Design review of the part shown in the three views and the two pictorial views. Dimensions are in mm from the part's minimum x, y and z. A direction names the side the tool comes from. Coordinates: 2 decimals unless noted, no trailing zeros. Loops run counter-clockwise (first coordinate to the right, second up) from the corner with the lowest first, then second, coordinate; pieces in that order, holes last. Notation, with made-up numbers: (-9, 24.5) -> (5, 24.5) arc R5 cw to (5, 33.5) -> close; hole circle Ø5 at (-29, -38). An arc over 180 degrees is marked (long way). Use CSV: the item, a comma, the result in double quotes.
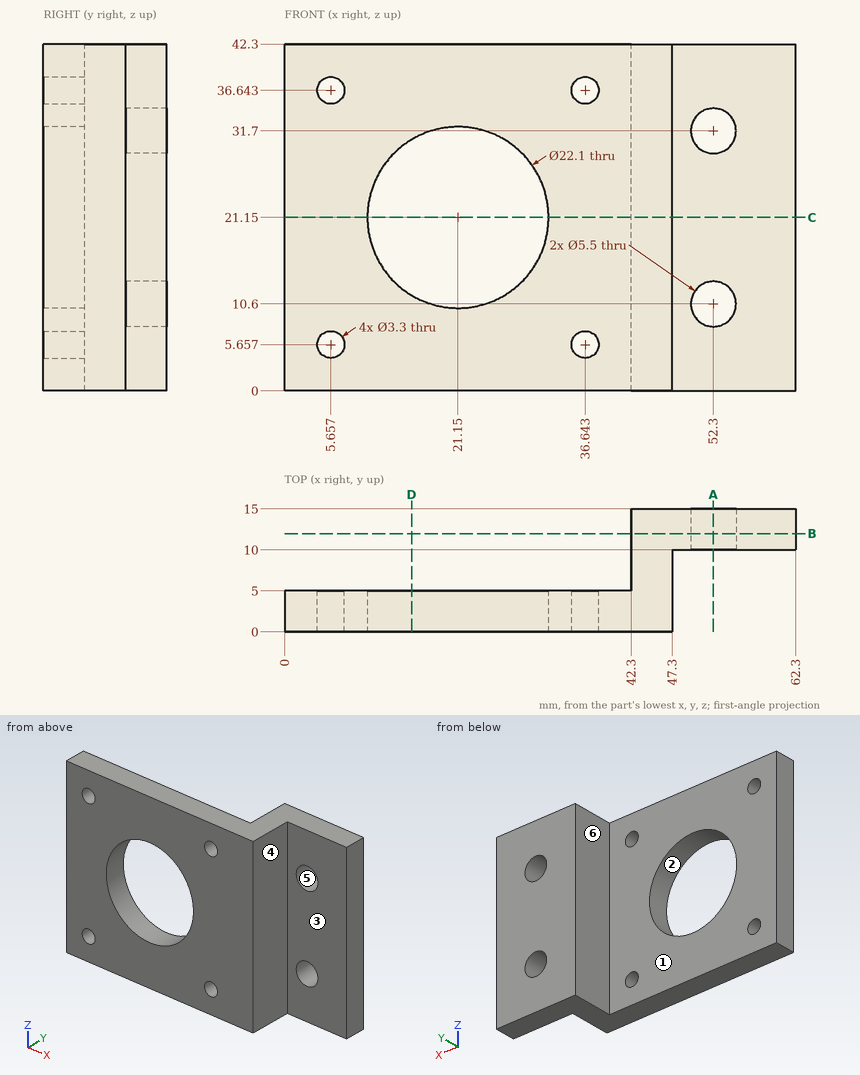
Item 1: Draft analysis for pull direction X (two halves, no side actions). For the marked faces 4, 5 and 6, state which applies: pulls with the +X half, pulls with the -X half, needs draft (parallel to the pull), parting line crosses it, or undercut.
Checked values:
face 4,"pulls with the +X half"
face 5,"undercut"
face 6,"pulls with the -X half"
Item 2: Add section C-C (z = 21.15). Give the boundary of the cut face in (x, y), then the cut area to 3 significant figures.
Checked values:
outline,"(0, 0) -> (10.1, 0) -> (10.1, 5) -> (0, 5) -> close; (32.2, 0) -> (47.3, 0) -> (47.3, 10) -> (62.3, 10) -> (62.3, 15) -> (42.3, 15) -> (42.3, 5) -> (32.2, 5) -> close"
area,"251 mm^2"
Item 3: Machinability: for the marked faces 1, 2 and 3, which of the approach directions +Z, -Z, +X, -X, +Y, -Y give a long, thin tool a straight path to every point of the face, cutting with its end or side? Answer none if there is none.
Checked values:
face 1,"+Z, -Z, -X, +Y"
face 2,"+Y, -Y"
face 3,"+Z, -Z, +X, -Y"
Item 4: Add section B-B (y = 12). Give the boundary of the cut face in (x, z).
Checked values:
outline,"(42.3, 0) -> (62.3, 0) -> (62.3, 42.3) -> (42.3, 42.3) -> close; hole circle Ø5.5 at (52.3, 10.6); hole circle Ø5.5 at (52.3, 31.7)"
Item 5: Add section A-A (x = 52.3). Give the boundary of the cut face in (y, z), then the cut area to 4 significant figures.
Checked values:
outline,"(10, 0) -> (15, 0) -> (15, 7.85) -> (10, 7.85) -> close; (10, 13.35) -> (15, 13.35) -> (15, 28.95) -> (10, 28.95) -> close; (10, 34.45) -> (15, 34.45) -> (15, 42.3) -> (10, 42.3) -> close"
area,"156.5 mm^2"
Item 6: Clearance check with flat-ended pins moving along their axes: pin 1 (5 mm diameter, centred on y = 4, z = 22.5, fed in from +X); pin 2 (8 mm diameter, centred on y = 9.5, z = 14.5, fed in from -X); pin 3 (2.5 mm diameter, centred on x = 5.66, z = 5.66, fed in from -Y); pin 4 (12 mm diameter, centred on x = 54.5, z = 17.5, fed in from -Y). State where each tip first meets the part, or that it passes through.
Checked values:
pin 1,"x = 47.3"
pin 2,"x = 42.3"
pin 3,"through"
pin 4,"y = 10"
Item 7: To check wall thickness, follow line 1 along Z through (x, y) = (52.3, 13.9); line 2 along X through (y, z) = (13.9, 31.7); line 3 along Y through (x, z) = (13, 10). State the ranges of each line that lie inside material, in increasing order.
Checked values:
line 1,"0 to 7.85, 13.35 to 28.95, 34.45 to 42.3"
line 2,"42.3 to 49.55, 55.05 to 62.3"
line 3,"0 to 5"
Item 8: Add section D-D (x = 15.5). Give the boundary of the cut face in (y, z), then the cut area to 3 significant figures.
Checked values:
outline,"(0, 0) -> (5, 0) -> (5, 11.65) -> (0, 11.65) -> close; (0, 30.65) -> (5, 30.65) -> (5, 42.3) -> (0, 42.3) -> close"
area,"117 mm^2"
